```python
from build123d import *

# Parameters (mm, degrees)
F0_W      = 170
F0_H      = 105
F0_R      = 2
F1_DEPTH  = 20
F2_DEPTH  = 15
F3_R      = 5
F4_R      = 3
F5_R      = 1
F6_R      = 3.1
F7_DEPTH  = 3.1
F8_R      = 3.1
F9_DEPTH  = 3.1
F10_R     = 3.1
F11_DEPTH = 3.1
F12_R     = 3.1
F13_DEPTH = 3.1
F14_DEPTH = 1
F15_ANGLE = 180


# Not quite as in the source:
# - a feature names something its author has since deleted; it is built from what else it names


with BuildPart() as f1:
    # F0 (on Top) → F1 (new body)
    with BuildSketch(Plane.XY):
        Rectangle(F0_W, F0_H)
        with Locations((0, -47.75)):
            Circle(F0_R, mode=Mode.SUBTRACT)
        with BuildLine():
            ThreePointArc((-75.5, 40), (-74.6213203436, 42.1213203436), (-72.5, 43))
            Line((-72.5, 43), (72.5, 43))
            ThreePointArc((72.5, 43), (74.6213203436, 42.1213203436), (75.5, 40))
            Line((75.5, 40), (75.5, -40))
            ThreePointArc((75.5, -40), (74.6213203436, -42.1213203436), (72.5, -43))
            Line((72.5, -43), (-72.5, -43))
            ThreePointArc((-72.5, -43), (-74.6213203436, -42.1213203436), (-75.5, -40))
            Line((-75.5, -40), (-75.5, 40))
        make_face(mode=Mode.SUBTRACT)
        with BuildLine():
            Line((72.5, 43), (-72.5, 43))
            ThreePointArc((-72.5, 43), (-74.6213203436, 42.1213203436), (-75.5, 40))
            Line((-75.5, 40), (-75.5, -40))
            ThreePointArc((-75.5, -40), (-74.6213203436, -42.1213203436), (-72.5, -43))
            Line((-72.5, -43), (72.5, -43))
            ThreePointArc((72.5, -43), (74.6213203436, -42.1213203436), (75.5, -40))
            Line((75.5, -40), (75.5, 40))
            ThreePointArc((75.5, 40), (74.6213203436, 42.1213203436), (72.5, 43))
        make_face()
        with Locations((0, -47.75)):
            Circle(F0_R)
    extrude(amount=F1_DEPTH)

    # F0 (on Top) → F2 (cut)
    with BuildSketch(Plane.XY):
        with BuildLine():
            Line((72.5, 43), (-72.5, 43))
            ThreePointArc((-72.5, 43), (-74.6213203436, 42.1213203436), (-75.5, 40))
            Line((-75.5, 40), (-75.5, -40))
            ThreePointArc((-75.5, -40), (-74.6213203436, -42.1213203436), (-72.5, -43))
            Line((-72.5, -43), (72.5, -43))
            ThreePointArc((72.5, -43), (74.6213203436, -42.1213203436), (75.5, -40))
            Line((75.5, -40), (75.5, 40))
            ThreePointArc((75.5, 40), (74.6213203436, 42.1213203436), (72.5, 43))
        make_face()
    extrude(amount=F2_DEPTH, mode=Mode.SUBTRACT)

    # F3
    f3_edges = [f1.edges().sort_by_distance(p)[0] for p in [
        (0, 52.5, 20),
        (-85, 0, 20),
        (0, -52.5, 20),
        (85, 0, 20),
        (85, 52.5, 10),
        (-85, 52.5, 10),
        (-85, -52.5, 10),
        (85, -52.5, 10),
    ]]
    fillet(f3_edges, radius=F3_R)

    # F4
    f4_edges = [f1.edges().sort_by_distance(p)[0] for p in [
        (0, 43, 15),
        (-74.62132, 42.12132, 15),
        (-75.5, 0, 15),
        (-74.62132, -42.12132, 15),
        (0, -43, 15),
        (74.62132, -42.12132, 15),
        (75.5, 0, 15),
        (74.62132, 42.12132, 15),
    ]]
    fillet(f4_edges, radius=F4_R)

    # F5
    f5_edges = [f1.edges().sort_by_distance(p)[0] for p in [
        (0, 52.5, 0),
        (83.535534, 51.035534, 0),
        (-83.535534, 51.035534, 0),
        (85, 0, 0),
        (-85, 0, 0),
        (83.535534, -51.035534, 0),
        (-83.535534, -51.035534, 0),
        (0, -52.5, 0),
        (0, 43, 0),
        (-74.62132, 42.12132, 0),
        (-75.5, 0, 0),
        (-74.62132, -42.12132, 0),
        (0, -43, 0),
        (74.62132, -42.12132, 0),
        (75.5, 0, 0),
        (74.62132, 42.12132, 0),
    ]]
    fillet(f5_edges, radius=F5_R)

    # F6 (on face) → F7 (cut)
    with BuildSketch(Plane.XZ.offset(52.5)):
        with Locations((42.5, 6)):
            Circle(F6_R)
        with Locations((-42.5, 6)):
            Circle(F6_R)
    extrude(amount=-F7_DEPTH, mode=Mode.SUBTRACT)

    # F8 (on face) → F9 (cut)
    with BuildSketch(Plane(origin=(0, 52.5, 0), x_dir=(-1, 0, 0), z_dir=(0, 1, 0))):
        with Locations((42.5, 6)):
            Circle(F8_R)
        with Locations((-42.5, 6)):
            Circle(F8_R)
    extrude(amount=-F9_DEPTH, mode=Mode.SUBTRACT)

    # F10 (on face) → F11 (cut)
    with BuildSketch(Plane(origin=(-85, 0, 0), x_dir=(0, -1, 0), z_dir=(-1, 0, 0))):
        with Locations((10, 6)):
            Circle(F10_R)
        with Locations((-10, 6)):
            Circle(F10_R)
    extrude(amount=-F11_DEPTH, mode=Mode.SUBTRACT)

    # F12 (on face) → F13 (cut)
    with BuildSketch(Plane.YZ.offset(85)):
        with Locations((10, 6)):
            Circle(F12_R)
        with Locations((-10, 6)):
            Circle(F12_R)
    extrude(amount=-F13_DEPTH, mode=Mode.SUBTRACT)

    # F0 (on Top) → F14 (cut)
    with BuildSketch(Plane.XY):
        with Locations((0, -47.75)):
            Circle(F0_R)
    extrude(amount=F14_DEPTH, mode=Mode.SUBTRACT)


with BuildPart() as f1_1:
    # F15: moved
    add(f1.part.rotate(Axis((0, 0, 0), (0, 1, 0)), F15_ANGLE))


solid = f1_1.part
```
Geometry: final body of the model. Coordinates: model frame, mm. A direction names the side the tool comes from. Coordinates: 2 decimals unless noted, no trailing zeros. Order: outer loops, then holes, each group sorted by start corner. A loop starts at its lowest first (then second) coordinate and runs counter-clockwise, first axis right, second up. Notation, with made-up numbers: (43.25, 89) - (97.25, 89) arc R19 ccw to (97.25, 104) - close; hole circle Ø11 at (47, 26.5). An arc over 180 degrees is marked (long way). Write each question's results on one line, items separated by ' | '.
(1) Set-up query: faces 5 (the face through (-42, -49.4, -6)), 6 (the face through (-83.47, 7.72, -8.1)), 7 (the face through (-43, 49.4, -6)), 8 (the face through (1, -43, -6)), 9 (the face through (81.9, -10, -6)). Return all of +Z, -Z, +X, -X, +Y, -Y with unobstructed straight access to the full face (end or side cutting, diameter ignored); none if empty.
Values found:
face 5: -Y | face 6: -X | face 7: +Y | face 8: +Z | face 9: +X
(2) Mould query, pull axis Z, two halves, no side actions, for faces 1 (the face through (-39.636, 50.972, -4.813)), 2 (the face through (0, -48, -1)), 3 (the face through (1, 1, -20)), 4 (the face through (43, -49.4, -6)). Classes: +Z half, -Z half, draft (parallel to the pull), parting line (faces both ways), or undercut.
Values found:
face 1: undercut | face 2: +Z half | face 3: -Z half | face 4: undercut
(3) Section query B-B, the plane x = 5. Return the cut outline in (y, z).
Values found:
outline: (-52.5, -15) arc R5 ccw to (-47.5, -20) - (47.5, -20) arc R5 ccw to (52.5, -15) - (52.5, -1) arc R1 ccw to (51.5, 0) - (44, 0) arc R1 ccw to (43, -1) - (43, -12) arc R3 cw to (40, -15) - (-40, -15) arc R3 cw to (-43, -12) - (-43, -1) arc R1 ccw to (-44, 0) - (-51.5, 0) arc R1 ccw to (-52.5, -1) - close
(4) First-contact query: pin 1 Ø7 at (y, z) = (-10, -6) entering from +X; pin 2 Ø3.5 at (y, z) = (-10, -6) entering from +X; pin 3 Ø1.9 at (x, z) = (-43, -7) entering from -Y; pin 4 Ø1.9 at (x, z) = (-43, -5.5) entering from +Y. Flat tips, straight axial feed; report the tip coordinate or a pass-through.
Values found:
pin 1: stops at x = 85 | pin 2: stops at x = 81.9 | pin 3: stops at y = -49.4 | pin 4: stops at y = 49.4
(5) Line query: line 1 (X direction, y = -21.5, z = -5.75); line 2 (Y direction, x = -70, z = -11.25); line 3 (Z direction, x = 15, y = -4.5). Output: solid intervals per line, ascending. Write a range as [from, to].
Values found:
line 1: x = [-85, -75.5], [75.5, 85] | line 2: y = [-52.5, -43], [43, 52.5] | line 3: z = [-20, -15]
(6) Section query A-A, the plane y = 37. Return the cut outline in (x, z), plus the area to 3 significant figures.
Values found:
outline: (-85, -15) arc R5 ccw to (-80, -20) - (80, -20) arc R5 ccw to (85, -15) - (85, -1) arc R1 ccw to (84, 0) - (76.5, 0) arc R1 ccw to (75.5, -1) - (75.5, -12) arc R3 cw to (72.5, -15) - (-72.5, -15) arc R3 cw to (-75.5, -12) - (-75.5, -1) arc R1 ccw to (-76.5, 0) - (-84, 0) arc R1 ccw to (-85, -1) - close | area: 1,130 mm²
(7) Section query C-C, the plane x = -42.5. Return the cut outline in (y, z), plus the area to 3 significant figures.
Values found:
outline: (-52.5, -15) arc R5 ccw to (-47.5, -20) - (47.5, -20) arc R5 ccw to (52.5, -15) - (52.5, -9.1) - (49.4, -9.1) - (49.4, -2.9) - (52.5, -2.9) - (52.5, -1) arc R1 ccw to (51.5, 0) - (44, 0) arc R1 ccw to (43, -1) - (43, -12) arc R3 cw to (40, -15) - (-40, -15) arc R3 cw to (-43, -12) - (-43, -1) arc R1 ccw to (-44, 0) - (-51.5, 0) arc R1 ccw to (-52.5, -1) - (-52.5, -2.9) - (-49.4, -2.9) - (-49.4, -9.1) - (-52.5, -9.1) - close | area: 764 mm²
(8) Section query D-D, the plane y = 10. Return the cut outline in (x, z), plus the area to 3 significant figures.
Values found:
outline: (-85, -15) arc R5 ccw to (-80, -20) - (80, -20) arc R5 ccw to (85, -15) - (85, -9.1) - (81.9, -9.1) - (81.9, -2.9) - (85, -2.9) - (85, -1) arc R1 ccw to (84, 0) - (76.5, 0) arc R1 ccw to (75.5, -1) - (75.5, -12) arc R3 cw to (72.5, -15) - (-72.5, -15) arc R3 cw to (-75.5, -12) - (-75.5, -1) arc R1 ccw to (-76.5, 0) - (-84, 0) arc R1 ccw to (-85, -1) - (-85, -2.9) - (-81.9, -2.9) - (-81.9, -9.1) - (-85, -9.1) - close | area: 1,090 mm²
